Here's how the part is built. I have some questions about the finished solid (model axes, mm). A direction names the side the tool comes from. Coordinates: 2 decimals unless noted, no trailing zeros. Write each loop counter-clockwise with the first axis right and the second up, starting at its lowest first coordinate (ties: lowest second). Pieces come first, ordered by that corner, then holes. Notation, with made-up numbers: M -30.5,68.25 L -9.5,68.25 A9 cw -9.5,83.25 Z; hole C 8.5,1.25 d11. An arc over 180 degrees is marked long. Write each question's results on one line, items separated by ' | '. Start each with the question number.
from build123d import *

# Parameters (mm, degrees)
SKETCH1_W           = 40
SKETCH1_H           = 44.45
SKETCH1_R           = 1.375
BOSS_EXTRUDE1_DEPTH = 4.7625
SKETCH2_W           = 40
SKETCH2_H           = 6.35
BOSS_EXTRUDE2_DEPTH = 20.066
SKETCH3_R           = 1.875
CUT_EXTRUDE1_DEPTH  = 27.416
FILLET1_R           = 6.35


with BuildPart() as part:
    # Sketch1 → Boss-Extrude1 (new body)
    with BuildSketch(Plane.XY):
        Rectangle(SKETCH1_W, SKETCH1_H)
        with Locations((-13, 15.958682008)):
            Circle(SKETCH1_R, mode=Mode.SUBTRACT)
        with Locations((13, 15.958682008)):
            Circle(SKETCH1_R, mode=Mode.SUBTRACT)
    extrude(amount=BOSS_EXTRUDE1_DEPTH)

    # Sketch2 → Boss-Extrude2 (add)
    with BuildSketch(Plane(origin=(0, 0, 0), x_dir=(-1, 0, 0), z_dir=(0, 0, -1))):
        with Locations((0, 1.016)):
            Rectangle(SKETCH2_W, SKETCH2_H)
    extrude(amount=BOSS_EXTRUDE2_DEPTH)

    # Sketch3 → Cut-Extrude1 (cut, through all)
    with BuildSketch(Plane(origin=(0, 4.191, 0), x_dir=(1, 0, 0), z_dir=(0, 1, 0))):
        with Locations((12.954, 10.033)):
            Circle(SKETCH3_R)
        with Locations((-12.954, 10.033)):
            Circle(SKETCH3_R)
    extrude(amount=-CUT_EXTRUDE1_DEPTH, mode=Mode.SUBTRACT)

    # Fillet1
    fillet1_edges = [part.edges().sort_by_distance(p)[0] for p in [
        (20, 1.016, -20.066),
        (-20, 1.016, -20.066),
        (20, -22.225, 2.38125),
        (-20, -22.225, 2.38125),
        (-20, 22.225, 2.38125),
        (20, 22.225, 2.38125),
    ]]
    fillet(fillet1_edges, radius=FILLET1_R)


solid = part.part
1) For pin 1 Ø14.5 at (x, y) = (9.5, 12.5) entering from -Z; pin 2 Ø6 at (x, z) = (4.5, -14) entering from -Y; pin 3 Ø6 at (x, z) = (1, -7.5) entering from +Y, each with a flat end and sliding along its axis, tell me the tip position at first contact or that it passes through.
2) I want a section at C-C, the plane y = -15. Write out the boundary of the cut face in (x, z).
3) Please list where these lines run through material, in increasing order: line 1 (X direction, y = 2.5, z = -8.5); line 2 (Y direction, x = 13, z = 1.75) (3 decimals); line 3 (Z direction, x = -8.5, y = -4). Write a range as [from, to].
4) We'd pull the mould along X, two halves only. Please class faces 4 (the flat face through (0, -22.225, 2)), 5 (the cylindrical face through (-18.189, 20.315, 2.415)), 6 (the cylindrical face through (-14, 16.9, 2.3)): pulls with the +X half, pulls with the -X half, needs draft (parallel to the pull), parting line crosses it, or undercut.
5) I want a section at D-D, the plane z = -6. Write out the boundary of the cut face in (x, y).
6) For faces 1 (the cylindrical face through (18.09, 1.06, -18.255)), 2 (the flat face through (0, 4.191, -10)), 3 (the flat face through (0, -2.159, -10)), which set-ups out of +Z, -Z, +X, -X, +Y, -Y let a thin tool reach every point of the face, with its end or its side?
7) I want a section at B-B, the plane x = -5. Write out the boundary of the cut face in (y, z) (1 decimal), then the cut area to 3 significant figures.
8) I want a section at A-A, the plane x = -13. Write out the boundary of the cut face in (y, z) (1 decimal).
Output:
1) pin 1: stops at z = 0 | pin 2: stops at y = -2.16 | pin 3: stops at y = 4.19
2) outline: M -20,0 L 20,0 L 20,4.76 L -20,4.76 Z
3) line 1: x = [-20, -14.03], [-11.87, 11.87], [14.03, 20] | line 2: y = [-22.225, 14.584], [17.334, 22.225] | line 3: z = [0, 4.76]
4) face 4: needs draft | face 5: pulls with the -X half | face 6: undercut
5) outline: M -20,-2.16 L 20,-2.16 L 20,4.19 L -20,4.19 Z
6) face 1: -Z, +X, +Y, -Y | face 2: -Z, +X, -X, +Y | face 3: -Z, +X, -X, -Y
7) outline: M -22.2,0 L -2.2,0 L -2.2,-20.1 L 4.2,-20.1 L 4.2,0 L 22.2,0 L 22.2,4.8 L -22.2,4.8 Z | area: 339 mm2
8) outline: M -22.2,0 L -2.2,0 L -2.2,-8.2 L 4.2,-8.2 L 4.2,0 L 14.6,0 L 14.6,4.8 L -22.2,4.8 Z; M -2.2,-20.1 L 4.2,-20.1 L 4.2,-11.9 L -2.2,-11.9 Z; M 17.3,0 L 22.2,0 L 22.2,4.8 L 17.3,4.8 Z
